Geometry check sheet. Reference: drawing and pictorial views, mm from the part's lowest x, y, z. A direction names the side the tool comes from. Round coordinates to 2 decimals unless told otherwise and drop trailing zeros. Order: outer loops, then holes, each group sorted by start corner. A loop starts at its lowest first (then second) coordinate and runs counter-clockwise, first axis right, second up.
(1) Sectioned sample at A-A (y = 13). Record the boundary of the cut face in (x, z), plus the area to 3 significant figures.
(2) Go/stop test with flat-tipped pins: pin 1 (2 mm diameter, centred on x = 41.5, y = 90.5, fed in from -Z); pin 2 (2 mm diameter, centred on y = 79.5, z = 8.5, fed in from +X); pin 3 (2 mm diameter, centred on x = 41, y = 59, fed in from -Z). Record where each tip stops, or that it passes through.
(3) Material ranges on line 1 along X through (y, z) = (17.5, 7) (1 decimal); line 2 along Y through (x, z) = (46.5, 6); line 3 along Z through (x, y) = (25.5, 10.5), recorded low to high.
(4) Set-up check for the marked faces 1, 2, 3 and 4: record each of +Z, -Z, +X, -X, +Y, -Y from which the full face is reachable in a straight line by a thin tool's end or side.
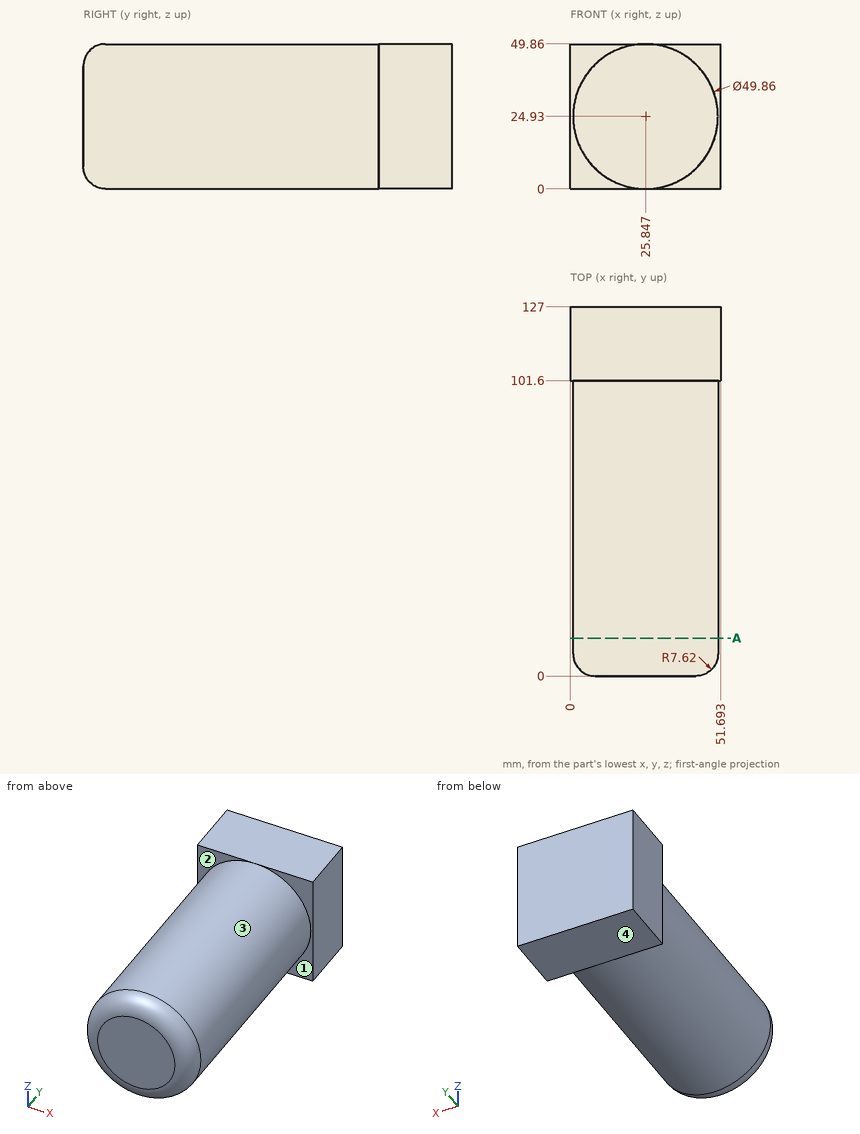
Answer below:
1. outline: circle Ø49.86 at (25.85, 24.93)
1. area: 1,950 mm2
2. pin 1: stops at z = 4.76
2. pin 2: stops at x = 45.43
2. pin 3: stops at z = 4.41
3. line 1: x = 8.5 to 43.2
3. line 2: y = 101.6 to 127
3. line 3: z = 0 to 49.86
4. face 1: +X, -Y
4. face 2: -X, -Y
4. face 3: -Y
4. face 4: -Z, +X, -X, +Y, -Y
